The listing builds one solid part. Answer for the finished solid, in the listing's coordinates (mm). Face numbers are marked on the shaded views. A direction names the side the tool comes from. Give positions to 0.01 mm unless a question says otherwise; leave off trailing zeros. Write each loop counter-clockwise with the first axis right and the second up, starting at its lowest first coordinate (ties: lowest second). Pieces come first, ordered by that corner, then holes. Notation, with made-up numbers: (38.25, 15) -> (79.25, 15) arc R19 cw to (79.25, 31) -> close; hole circle Ø6 at (17.25, 89). An arc over 180 degrees is marked (long way). Use CSV: the item, a comma, the result in double quotes. Start each with the question number.
Autodesk Inventor part; units mm, degrees
ref_plane "Plano de trabajo1" through (0, 25, 0) normal (0, 1, 0) x (1, 0, 0)
ref_plane "YZ Plane" through (0, 0, 0) normal (1, 0, 0) x (0, 1, 0)
ref_plane "XZ Plane" through (0, 0, 0) normal (0, 1, 0) x (-1, 0, 0)
sketch "Boceto1" plane through (0, 0, 0) normal (0, 1, 0) x (-1, 0, 0)
  line L0 (-25, 75) -> (25, 75)
  line L1 (25, 75) -> (25, -75)
  line L2 (25, -75) -> (-25, -75)
  line L3 (-25, -75) -> (-25, 75)
  line L4 (-25, 75) -> (25, -75) construction
  line L5 (25, 75) -> (-25, -75) construction
  point P0 (0, 0)
  dimension "d0" = 50
  dimension "d1" = 150
extrude "Extrusión1" add sketch "Boceto1" along normal blind 50
sketch "Boceto2" plane through (25, 0, -75) normal (0, 0, -1) x (-1, 0, 0)
  line L0 (50, 50) -> (0, 50)
  line L1 (50, 50) -> (80, 50)
  line L2 (0, 0) -> (50, 0)
  line L3 (50, 0) -> (80, 0)
  arc A0 (80, 0) -> (80, 50) centre (78.3333, 25) ccw
  line L4 (50, 0) -> (50, 50)
  line L5 (50, 50) -> (50, 0)
  point P0 (25, 0)
  dimension "d4" = 30
  dimension "d5" = 30
extrude "Extrusión2" add sketch "Boceto2" against normal blind 10
ref_plane "Plano de trabajo1" through (0, 25, 0) normal (0, 1, 0) x (1, 0, 0)
sketch "Boceto3" plane through (25, 0, -75) normal (0, 0, -1) x (-1, 0, 0)
  point P0 (25, 0)
  point P1 (84.2508, 24.8764)
hole "Agujero1" at (-59.2508, 24.8764, -75) direction (0, 0, 1) diameter 15 end through all
sketch "Boceto4" plane through (-25, 0, 75) normal (0, 0, 1) x (1, 0, 0)
  arc A0 (-30, 50) -> (-30, 0) centre (-28.3333, 25) ccw
  line L0 (0, 50) -> (-30, 50)
  line L1 (-30, 0) -> (0, 0)
  line L2 (0, 0) -> (0, 50)
  point P0 (25, 0)
extrude "Extrusión3" add sketch "Boceto4" against normal blind 10
sketch "Boceto5" plane through (25, 0, 75) normal (0, 0, 1) x (1, 0, 0)
  point P0 (-25, 0)
  point P1 (-83.9488, 24.8764)
hole "Agujero2" at (-58.9488, 24.8764, 75) direction (0, 0, -1) diameter 15 end through all
sketch "Boceto6" plane through (25, 0, 75) normal (1, 0, 0) x (0, 0, -1)
  point P0 (75, 0)
shell "Vaciado1" thickness 5 removed faces 1 at (25, 16.6667, -25)
sketch "Boceto7" plane through (-25, 0, -65) normal (-1, 0, 0) x (0, 0, 1)
  point P0 (65, 0)
  point P1 (65.2039, 25.1019)
hole "Agujero3" at (-25, 25.1019, 0.2039) direction (1, 0, 0) diameter 40.24 end through all
properties part number "primer rotor"
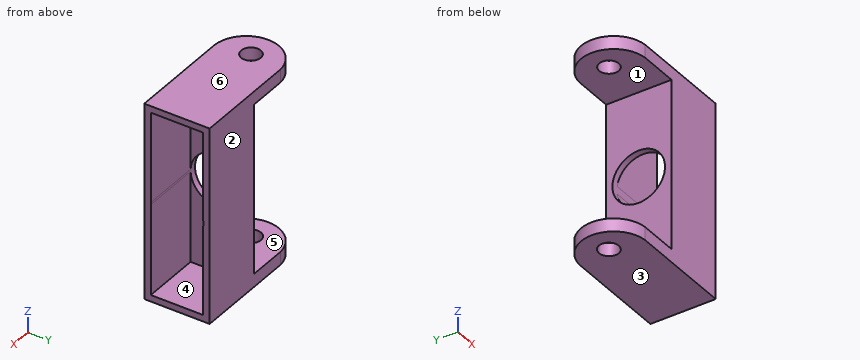
Q1. Section D-D on z = 32 is taken. Give the vertices of the cut face in (x, y).
Q2. The mould has two halves that part along Z. Classify the marked faces 1, 2 and 3: +Z half, -Z half, draft (parallel to the pull), parting line (faces both ways), or undercut.
Q3. Flat-ended cylindrical pins translate along their axes: pin 1 Ø25 at (y, z) = (18.5, 12.5) entering from -X; pin 2 Ø1 at (y, z) = (42.5, -35.5) entering from +X. Find the tip coordinate at first contact, or state that the pin passes through.
Q4. For the marked faces 4, 5 and 6, determine the directions among +Z, -Z, +X, -X, +Y, -Y from which every point of the face is accessible in a straight line to the end or side of a thin tool.
Q5. Section B-B on y = 34 is taken. Give the vertices of the cut face in (x, z).
Q6. Section C-C on z = -9 is taken. Give the vertices of the cut face in (x, y).
Q7. Straight lines are drawn through the part: L1, parallel to Z at x = -54, y = 14.5; L2, parallel to Y at x = 14.5, z = 58; L3, parallel to Z at x = 2, y = 31. For each, find the intervals that lie inside material, in ascending order.
Q8. Section A-A on x = -46.5 is taken. Give the vertices of the cut face in (y, z), then the cut area to 3 significant figures.
Output:
1,outline,"(-25, 0) -> (25, 0) -> (25, 5) -> (-20, 5) -> (-20, 45) -> (25, 45) -> (25, 50) -> (-25, 50) -> close"
2,face 1,"undercut"
2,face 2,"draft"
2,face 3,"-Z half"
3,pin 1,"x = -25"
3,pin 2,"x = -20"
4,face 4,"+X"
4,face 5,"-X, +Y, -Y"
4,face 6,"+Z, +X, -X, +Y, -Y"
5,outline,"(-76.72, -75) -> (25, -75) -> (25, -70) -> (-20, -70) -> (-20, -17.84) -> (-25, -17.84) -> (-25, -65) -> (-76.72, -65) -> close; (-76.72, 65) -> (-25, 65) -> (-25, 18.25) -> (-20, 18.25) -> (-20, 70) -> (25, 70) -> (25, 75) -> (-76.72, 75) -> close"
6,outline,"(-25, 0) -> (25, 0) -> (25, 5) -> (-20, 5) -> (-20, 7.21) -> (-25, 7.21) -> close; (-25, 42.99) -> (-20, 42.99) -> (-20, 45) -> (25, 45) -> (25, 50) -> (-25, 50) -> close"
7,L1,"-75 to -65, 65 to 75"
7,L2,"0 to 5, 45 to 50"
7,L3,"-75 to -70, 70 to 75"
8,outline,"(0, -75) -> (50, -75) -> (50, -65) -> (0, -65) -> close; (0, 65) -> (50, 65) -> (50, 75) -> (0, 75) -> close"
8,area,"1,000 mm²"
